The listing builds one solid part. Answer for the finished solid, in the listing's coordinates (mm). Face numbers are marked on the shaded views. A direction names the side the tool comes from. Give positions to 0.01 mm unless a question says otherwise; leave off trailing zeros. Write each loop counter-clockwise with the first axis right and the second up, starting at its lowest first coordinate (ties: lowest second). Pieces come first, ordered by that corner, then holes. Notation, with made-up numbers: (78, 32.25) -> (136, 32.25) arc R25 cw to (136, 47.25) -> close; hole circle Ø8 at (68, 71). An arc over 180 degrees is marked (long way). One line per question, with ' | ' between items.
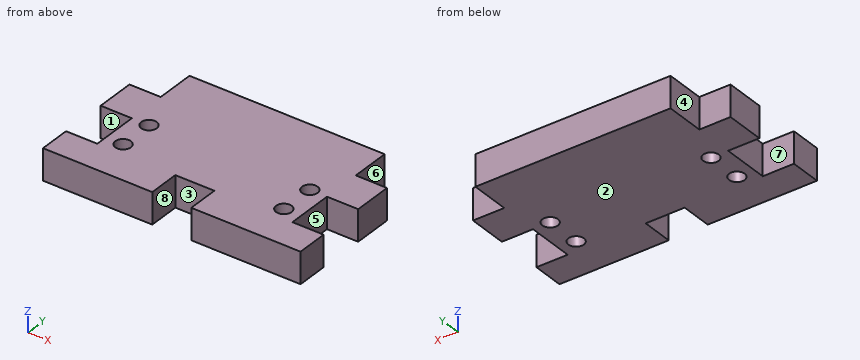
from build123d import *

# Parameters (mm, degrees)
SKETCH_1_W          = 33
SKETCH_1_H          = 20
EXTRUDE_1_DEPTH     = 4
SKETCH_2_W          = 4
SKETCH_2_H          = 5
SKETCH_2_H_2        = 6
SKETCH_2_W_2        = 5
SKETCH_2_H_3        = 4
CUT_EXTRUDE_1_DEPTH = 4
SKETCH_3_R          = 1
CUT_EXTRUDE_2_DEPTH = 4


with BuildPart() as part:
    # Эскиз1 → Бобышка-Вытянуть1 (new body)
    with BuildSketch(Plane.XY):
        with Locations((16.5, 10)):
            Rectangle(SKETCH_1_W, SKETCH_1_H)
    extrude(amount=EXTRUDE_1_DEPTH)

    # Эскиз2 → Вырез-Вытянуть1 (cut)
    with BuildSketch(Plane(origin=(0, 0, 0), x_dir=(-1, 0, 0), z_dir=(0, 0, -1))):
        with Locations((-2, 17.5)):
            Rectangle(SKETCH_2_W, SKETCH_2_H)
        with Locations((-2, 7)):
            Rectangle(SKETCH_2_W, SKETCH_2_H_2)
        with Locations((-16.5, 2)):
            Rectangle(SKETCH_2_W_2, SKETCH_2_H_3)
        with Locations((-31, 7)):
            Rectangle(SKETCH_2_W, SKETCH_2_H_2)
        with Locations((-31, 17.5)):
            Rectangle(SKETCH_2_W, SKETCH_2_H)
    extrude(amount=-CUT_EXTRUDE_1_DEPTH, mode=Mode.SUBTRACT)

    # Эскиз3 → Вырез-Вытянуть2 (cut)
    with BuildSketch(Plane.XY.offset(4)):
        with Locations((6.2, 10)):
            Circle(SKETCH_3_R)
        with Locations(Location((26.8, 10, 0), (0, 0, 180))):
            Circle(SKETCH_3_R)
        with Locations((6.2, 5.5)):
            Circle(SKETCH_3_R)
        with Locations(Location((26.8, 5.5, 0), (0, 0, 180))):
            Circle(SKETCH_3_R)
    extrude(amount=-CUT_EXTRUDE_2_DEPTH, mode=Mode.SUBTRACT)


solid = part.part
Item 1: Find section A-A (y = 5.5). Write down the section's boundary in (x, z).
Answers below:
outline: (4, 0) -> (5.2, 0) -> (5.2, 4) -> (4, 4) -> close; (7.2, 0) -> (25.8, 0) -> (25.8, 4) -> (7.2, 4) -> close; (27.8, 0) -> (29, 0) -> (29, 4) -> (27.8, 4) -> close
Item 2: Find section C-C (z = 1.75). Write down the section's boundary in (x, y), then the cut area to 3 significant figures.
Answers below:
outline: (0, 0) -> (14, 0) -> (14, 4) -> (19, 4) -> (19, 0) -> (33, 0) -> (33, 4) -> (29, 4) -> (29, 10) -> (33, 10) -> (33, 15) -> (29, 15) -> (29, 20) -> (4, 20) -> (4, 15) -> (0, 15) -> (0, 10) -> (4, 10) -> (4, 4) -> (0, 4) -> close; hole circle Ø2 at (6.2, 5.5); hole circle Ø2 at (6.2, 10); hole circle Ø2 at (26.8, 5.5); hole circle Ø2 at (26.8, 10) | area: 539 mm²
Item 3: Find section D-D (y = 7.75). Write down the section's boundary in (x, z), then the cut area to 3 significant figures.
Answers below:
outline: (4, 0) -> (29, 0) -> (29, 4) -> (4, 4) -> close | area: 100 mm²
Item 4: Consider line 1 (Y direction, x = 6.2, z = 2.95); line 2 (Y direction, x = 31, z = 1.85); line 3 (Y direction, x = 7, z = 1.75). Determine where each line is inside the solid, lowest interval first. Write a range as [from, to].
Answers below:
line 1: [0, 4.5], [6.5, 9], [11, 20] | line 2: [0, 4], [10, 15] | line 3: [0, 4.9], [6.1, 9.4], [10.6, 20]
Item 5: Flat-ended cylindrical pins translate along their axes: pin 1 (2 mm diameter, centred on y = 16.5, z = 1.5, fed in from +X); pin 2 (1.2 mm diameter, centred on x = 6.2, y = 5.5, fed in from -Z); pin 3 (1.2 mm diameter, centred on y = 16.5, z = 2, fed in from -X); pin 4 (1.2 mm diameter, centred on x = 15.5, z = 2, fed in from -Y). Find the tip coordinate at first contact, or state that the pin passes through.
Answers below:
pin 1: x = 29 | pin 2: through | pin 3: x = 4 | pin 4: y = 4
Item 6: Determine the mould class of the marked faces 1, 2 and 3 for opening direction Y: pulls with the +Y half, pulls with the -Y half, needs draft (parallel to the pull), parting line crosses it, or undercut.
Answers below:
face 1: undercut | face 2: needs draft | face 3: pulls with the -Y half
Item 7: Find section B-B (x = 26.8). Write down the section's boundary in (y, z).
Answers below:
outline: (0, 0) -> (4.5, 0) -> (4.5, 4) -> (0, 4) -> close; (6.5, 0) -> (9, 0) -> (9, 4) -> (6.5, 4) -> close; (11, 0) -> (20, 0) -> (20, 4) -> (11, 4) -> close
Item 8: A tool of negligible diameter and unlimited length cuts with its end or side. For the marked faces 4, 5, 6, 7 and 8, from which of +Z, -Z, +X, -X, +Y, -Y can it reach the whole face along a straight path? Write none if from no direction.
Answers below:
face 4: +Z, -Z, -X, +Y | face 5: +Z, -Z, +X | face 6: +Z, -Z, +X, +Y | face 7: +Z, -Z, -X | face 8: +Z, -Z, -Y
